from build123d import *

# Parameters (mm, degrees)
AUFSATZ_LINEAR_AUSTRAGEN1_DEPTH  = 20
SCHNITT_LINEAR_AUSTRAGEN2_REACH  = 24.753
SKIZZE8_W                        = 11
SKIZZE8_H                        = 5
AUFSATZ_LINEAR_AUSTRAGEN3_DEPTH  = 8.34
SCHNITT_LINEAR_AUSTRAGEN3_REACH  = 28.626
SKIZZE12_W                       = 1.5
SKIZZE12_H                       = 2
AUFSATZ_LINEAR_AUSTRAGEN4_DEPTH  = 3.98
AUFSATZ_LINEAR_AUSTRAGEN5_DEPTH  = 2.67
AUFSATZ_LINEAR_AUSTRAGEN6_DEPTH  = 2.67
SCHNITT_LINEAR_AUSTRAGEN4_REACH  = 43.942
SKIZZE17_W                       = 3
SKIZZE17_H                       = 16.288675134
AUFSATZ_LINEAR_AUSTRAGEN15_DEPTH = 6.65


with BuildPart() as part:
    # Skizze1 → Aufsatz-Linear austragen1 (new body)
    with BuildSketch(Plane(origin=(0, 0, 0), x_dir=(1, 0, 0), z_dir=(0, 1, 0))):
        Polygon((5.5, -4.17), (-5.5, -4.17), (-5.5, -1.5), (-7.5, -1.5), (-7.5, 1.5), (-5.5, 1.5), (-5.5, 4.17), (5.5, 4.17), (5.5, 1.5), (7.5, 1.5), (7.5, -1.5), (5.5, -1.5), align=None)
        Polygon((-5, 1), (-5, 3.67), (5, 3.67), (5, 1), (7, 1), (7, -1), (5, -1), (5, -3.67), (-5, -3.67), (-5, -1), (-7, -1), (-7, 1), align=None, mode=Mode.SUBTRACT)
    extrude(amount=AUFSATZ_LINEAR_AUSTRAGEN1_DEPTH)

    # Skizze8 → Schnitt-Linear austragen2 (cut, up to next)
    with BuildSketch(Plane(origin=(0, 0, 3.67), x_dir=(-1, 0, 0), z_dir=(0, 0, -1)), mode=Mode.PRIVATE) as schnitt_linear_austragen2_sk1:
        with Locations((0, 2.5)):
            Rectangle(SKIZZE8_W, SKIZZE8_H)
    schnitt_linear_austragen2_tool1 = extrude(schnitt_linear_austragen2_sk1.sketch, amount=-SCHNITT_LINEAR_AUSTRAGEN2_REACH, mode=Mode.PRIVATE) & part.part
    add(schnitt_linear_austragen2_tool1.solids().sort_by_distance((0, 2.5, 3.67))[0], mode=Mode.SUBTRACT)

    # Skizze10 → Aufsatz-Linear austragen3 (add)
    with BuildSketch(Plane(origin=(0, 0, -4.17), x_dir=(-1, 0, 0), z_dir=(0, 0, -1))):
        Polygon((5.5, 20), (7.211324865, 20), (17.211324865, 37.320508076), (17.644337567, 37.070508076), (7.5, 19.5), (5.5, 19.5), align=None)
    extrude(amount=-AUFSATZ_LINEAR_AUSTRAGEN3_DEPTH)

    # Skizze12 → Schnitt-Linear austragen3 (cut, up to next)
    with BuildSketch(Plane.XZ.offset(-19.5), mode=Mode.PRIVATE) as schnitt_linear_austragen3_sk1:
        with Locations((-6.25, 0)):
            Rectangle(SKIZZE12_W, SKIZZE12_H)
    schnitt_linear_austragen3_tool1 = extrude(schnitt_linear_austragen3_sk1.sketch, amount=-SCHNITT_LINEAR_AUSTRAGEN3_REACH, mode=Mode.PRIVATE) & part.part
    add(schnitt_linear_austragen3_tool1.solids().sort_by_distance((-6.25, 19.5, 0))[0], mode=Mode.SUBTRACT)

    # Skizze13 → Aufsatz-Linear austragen4 (add)
    with BuildSketch(Plane(origin=(0, 0, -4.17), x_dir=(-1, 0, 0), z_dir=(0, 0, -1))):
        Polygon((17.211324865, 37.320508076), (9.561324865, 24.070319398), (9.994337567, 23.820319398), (17.644337567, 37.070508076), align=None)
    aufsatz_linear_austragen4 = extrude(amount=AUFSATZ_LINEAR_AUSTRAGEN4_DEPTH)

    # Skizze15 → Aufsatz-Linear austragen5 (add)
    with BuildSketch(Plane(origin=(0, 0, -1.5), x_dir=(-1, 0, 0), z_dir=(0, 0, -1))):
        Polygon((5.5, 8), (5.5, 19.5), (7.5, 19.5), (17.644337567, 37.070508076), (7.5, 8), align=None)
    extrude(amount=AUFSATZ_LINEAR_AUSTRAGEN5_DEPTH)

    # Spiegeln1: Aufsatz-Linear austragen4 across plane
    add(aufsatz_linear_austragen4.mirror(Plane.XY))

    # Skizze16 → Aufsatz-Linear austragen6 (add)
    with BuildSketch(Plane.XY.offset(1.5)):
        Polygon((-17.644337567, 37.070508076), (-7.5, 8), (-5.5, 8), (-5.5, 19.5), (-7.5, 19.5), align=None)
    extrude(amount=AUFSATZ_LINEAR_AUSTRAGEN6_DEPTH)

    # Skizze17 → Schnitt-Linear austragen4 (cut, up to next)
    with BuildSketch(Plane(origin=(2.818747687, 1.627404736, 0), x_dir=(0, 0, 1), z_dir=(-0.8660254037844417, -0.49999999999999467, 0)), mode=Mode.PRIVATE) as schnitt_linear_austragen4_sk1:
        with Locations((0, 28.781832941)):
            Rectangle(SKIZZE17_W, SKIZZE17_H)
    schnitt_linear_austragen4_tool1 = extrude(schnitt_linear_austragen4_sk1.sketch, amount=-SCHNITT_LINEAR_AUSTRAGEN4_REACH, mode=Mode.PRIVATE) & part.part
    add(schnitt_linear_austragen4_tool1.solids().sort_by_distance((-11.572169, 26.553203, 0))[0], mode=Mode.SUBTRACT)

    # Skizze22 → Aufsatz-Linear austragen15 (add)
    with BuildSketch(Plane.XY.offset(-1.5)):
        Polygon((-17.611390326, 36.976091556), (-12.603409607, 22.624780496), (-13.075492208, 22.460044288), (-18.083472926, 36.811355348), align=None)
    aufsatz_linear_austragen15 = extrude(amount=-AUFSATZ_LINEAR_AUSTRAGEN15_DEPTH)

    # Spiegeln2: Aufsatz-Linear austragen15 across plane
    add(aufsatz_linear_austragen15.mirror(Plane.XY))


solid = part.part
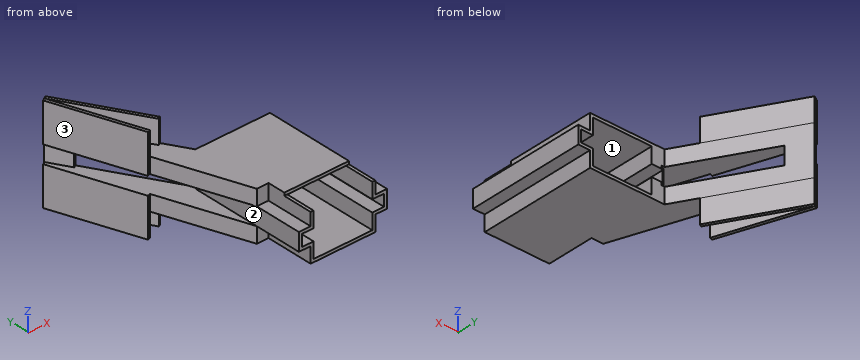
Geometry check sheet. Reference: the model listing, model coordinates, mm. Face numbers are marked on the shaded views. A direction names the side the tool comes from. Give positions to 0.01 mm unless a question says otherwise; leave off trailing zeros. Order: outer loops, then holes, each group sorted by start corner. A loop starts at its lowest first (then second) coordinate and runs counter-clockwise, first axis right, second up. Notation, with made-up numbers: (10, 87.5) - (33, 87.5) arc R22 cw to (33, 123.5) - close; hole circle Ø5 at (70.5, 61.25). An arc over 180 degrees is marked (long way). Answer as a JSON object with one key per item and string values.
(1) Depth check by flat-ended pin: pin 1 Ø3 at (y, z) = (25.5, 6.5) entering from -X; pin 2 Ø1 at (y, z) = (9.5, 0) entering from -X; pin 3 Ø8 at (y, z) = (28, -1.5) entering from +X. Enter the tip coordinate at first touch or a pass-through.
Report:
{"pin 1": "x = -14.66", "pin 2": "x = -7.5", "pin 3": "x = -9.52"}
(2) Tool access check on the marked faces 1, 2 and 3. Record the directions out of +Z, -Z, +X, -X, +Y, -Y that give a thin tool (end or side, any length) a straight path to the whole face; none if there is none.
Report:
{"face 1": "+Y, -Y", "face 2": "-X, +Y, -Y", "face 3": "+Z, -Z, -X, -Y"}
(3) Cross-section at C-C (x = -2.25). Record the cut outline in (y, z), then the cut area to 3 significant figures.
Report:
{"outline": "(0, -4.17) - (20, -4.17) - (20, -3.67) - (0, -3.67) - close; (5, 3.67) - (20, 3.67) - (20, 4.17) - (5, 4.17) - close", "area": "17.5 mm^2"}
(4) Cross-section at B-B (y = 5.5). Record the cut outline in (x, z), then the cut area to 3 significant figures.
Report:
{"outline": "(-7.5, -1.5) - (-5.5, -1.5) - (-5.5, -4.17) - (5.5, -4.17) - (5.5, -1.5) - (7.5, -1.5) - (7.5, 1.5) - (5.5, 1.5) - (5.5, 4.17) - (-5.5, 4.17) - (-5.5, 1.5) - (-7.5, 1.5) - close; hole (-7, -1) - (-5, -1) - (-5, -3.67) - (5, -3.67) - (5, -1) - (7, -1) - (7, 1) - (5, 1) - (5, 3.67) - (-5, 3.67) - (-5, 1) - (-7, 1) - close", "area": "22.3 mm^2"}
(5) Cross-section at A-A (z = 0). Record the cut outline in (x, y), then the cut area to 3 significant figures.
Report:
{"outline": "(-17.64, 37.07) - (-15.64, 33.61) - (-15.21, 33.86) - (-17.21, 37.32) - close; (-7.5, 0) - (-7, 0) - (-7, 19.79) - (-7.5, 19.5) - close; (7, 0) - (7.5, 0) - (7.5, 20) - (7, 20) - close", "area": "21.8 mm^2"}
(6) Material ranges on line 1 (Z direction, x = -1.5, y = 6); line 2 (Z direction, x = -14, y = 28.5); line 3 (X direction, y = 18, z = 0), recorded low to high.
Report:
{"line 1": "-4.17 to -3.67, 3.67 to 4.17", "line 2": "-4.17 to -1.5, 1.5 to 4.17", "line 3": "-7.5 to -7, 7 to 7.5"}
(7) Cross-section at D-D (z = -2.25). Record the cut outline in (x, y).
Report:
{"outline": "(-18.08, 36.81) - (-13.08, 22.46) - (-12.6, 22.62) - (-7.5, 8) - (-5.5, 8) - (-5.5, 0) - (-5, 0) - (-5, 20) - (-7.21, 20) - (-17.21, 37.32) - (-17.64, 37.07) - (-17.61, 36.98) - close; (5, 0) - (5.5, 0) - (5.5, 20) - (5, 20) - close"}
